Can you work these out from the model? Positions are in its coordinate system, mm. Face numbers are marked on the shaded views. A direction names the side the tool comes from. Give positions to 0.01 mm unless a question says otherwise; leave off trailing zeros. Loops run counter-clockwise (first coordinate to the right, second up) from the corner with the lowest first, then second, coordinate; pieces in that order, holes last. Notation, with made-up numbers: M 4,27 L 47,27 A32 cw 47,58 Z; hole C -18.5,21 d8. An arc over 180 degrees is marked long. Answer as a JSON object with one key per item and string values.
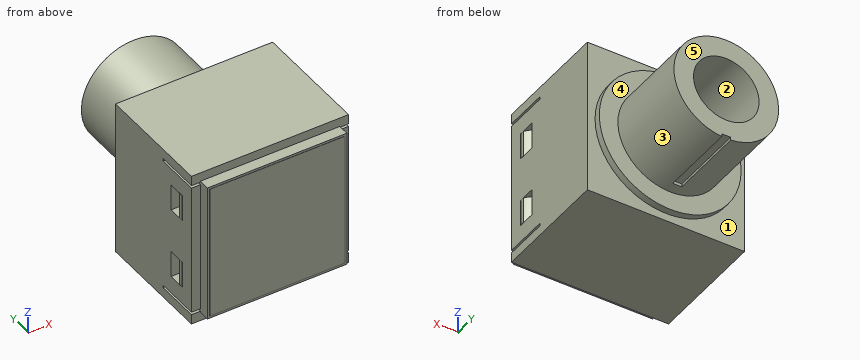
Autodesk Inventor part; units mm, degrees
ref_plane "body_to_dummy_XY" through (0, 0, 0) normal (0, 1, 0) x (1, 0, 0)
ref_plane "body_to_dummy_YZ" through (0, 0, 0) normal (1, 0, 0) x (0, 0, -1)
ref_plane "body_to_dummy_ZX" through (0, 0, 0) normal (0, 0, -1) x (0, 1, 0)
sketch "Sketch_1" plane through (0, 0, 0) normal (1, 0, 0) x (0, 1, 0)
  line L0 (0, 9.0043) -> (-15.5956, 9.0043)
  line L1 (-15.5956, 9.0043) -> (-15.5956, -9.0043)
  line L2 (-15.5956, -9.0043) -> (0, -9.0043)
  line L3 (0, -9.0043) -> (0, 9.0043)
extrude "Extrusion1" add sketch "Sketch_1" along normal mid plane 18.0086
sketch "Sketch_2" plane through (0, 0, 0) normal (0, 1, 0) x (-1, 0, 0)
  line L0 (12.2936, -12.2936) -> (12.2936, 12.2936)
  line L1 (12.2936, 12.2936) -> (-12.2936, 12.2936)
  line L2 (-12.2936, 12.2936) -> (-12.2936, -12.2936)
  line L3 (-12.2936, -12.2936) -> (12.2936, -12.2936)
  circle A0 centre (0, 0) radius 8.128
extrude "Extrusion2" cut sketch "Sketch_2" along normal mid plane 1.524
sketch "Sketch_3" plane through (0, -15.5956, 0) normal (0, 1, 0) x (1, 0, 0)
  line L0 (-11.5316, 11.5316) -> (-11.5316, -11.5316)
  line L1 (-11.5316, -11.5316) -> (11.5316, -11.5316)
  line L2 (11.5316, -11.5316) -> (11.5316, 11.5316)
  line L3 (11.5316, 11.5316) -> (-11.5316, 11.5316)
  line L4 (-7.9883, 7.9883) -> (-7.9883, -7.9883)
  line L5 (-7.9883, -7.9883) -> (7.9883, -7.9883)
  line L6 (7.9883, -7.9883) -> (7.9883, 7.9883)
  line L7 (7.9883, 7.9883) -> (-7.9883, 7.9883)
extrude "Extrusion3" cut sketch "Sketch_3" along normal mid plane 2.54
sketch "Sketch_4" plane through (0, -14.3256, 0) normal (0, 1, 0) x (1, 0, 0)
  line L0 (-12.446, 12.446) -> (-12.446, -12.446)
  line L1 (-12.446, -12.446) -> (12.446, -12.446)
  line L2 (12.446, -12.446) -> (12.446, 12.446)
  line L3 (12.446, 12.446) -> (-12.446, 12.446)
  line L4 (-11.5316, -7.5692) -> (-7.9883, -7.5692)
  line L5 (-7.9883, -7.5692) -> (-7.9883, -7.874)
  line L6 (-7.9883, -7.874) -> (-11.5316, -7.874)
  line L7 (-11.5316, -7.874) -> (-11.5316, -11.5316)
  line L8 (-11.5316, -11.5316) -> (11.5316, -11.5316)
  line L9 (11.5316, -11.5316) -> (11.5316, -7.874)
  line L10 (11.5316, -7.874) -> (7.9883, -7.874)
  line L11 (7.9883, -7.874) -> (7.9883, -7.5692)
  line L12 (7.9883, -7.5692) -> (11.5316, -7.5692)
  line L13 (11.5316, -7.5692) -> (11.5316, 7.5692)
  line L14 (11.5316, 7.5692) -> (7.9883, 7.5692)
  line L15 (7.9883, 7.5692) -> (7.9883, 7.874)
  line L16 (7.9883, 7.874) -> (11.5316, 7.874)
  line L17 (11.5316, 7.874) -> (11.5316, 11.5316)
  line L18 (11.5316, 11.5316) -> (-11.5316, 11.5316)
  line L19 (-11.5316, 11.5316) -> (-11.5316, 7.874)
  line L20 (-11.5316, 7.874) -> (-7.9883, 7.874)
  line L21 (-7.9883, 7.874) -> (-7.9883, 7.5692)
  line L22 (-7.9883, 7.5692) -> (-11.5316, 7.5692)
  line L23 (-11.5316, 7.5692) -> (-11.5316, -7.5692)
extrude "Extrusion4" cut sketch "Sketch_4" along normal mid plane 10.16
sketch "Sketch_5" plane through (0, -14.3256, 0) normal (0, 1, 0) x (1, 0, 0)
  line L0 (-7.7343, 7.7343) -> (-7.7343, -7.7343)
  line L1 (-7.7343, -7.7343) -> (7.7343, -7.7343)
  line L2 (7.7343, -7.7343) -> (7.7343, 7.7343)
  line L3 (7.7343, 7.7343) -> (-7.7343, 7.7343)
extrude "Extrusion5" add sketch "Sketch_5" against normal blind 1.2954
sketch "Sketch_6" plane through (9.0043, 0, 0) normal (1, 0, 0) x (0, 0, -1)
  line L0 (2.54, -10.668) -> (2.54, -12.7)
  line L1 (2.54, -12.7) -> (5.588, -12.7)
  line L2 (5.588, -12.7) -> (5.588, -10.668)
  line L3 (5.588, -10.668) -> (2.54, -10.668)
extrude "Extrusion6" cut sketch "Sketch_6" against normal blind 18.0086
sketch "Sketch_7" plane through (9.0043, 0, 0) normal (1, 0, 0) x (0, 0, -1)
  line L0 (-5.588, -10.668) -> (-5.588, -12.7)
  line L1 (-5.588, -12.7) -> (-2.54, -12.7)
  line L2 (-2.54, -12.7) -> (-2.54, -10.668)
  line L3 (-2.54, -10.668) -> (-5.588, -10.668)
extrude "Extrusion7" cut sketch "Sketch_7" against normal blind 18.0086
sketch "Sketch_8" plane through (0, 0, 4.064) normal (0, 0, 1) x (1, 0, 0)
  line L0 (-9.0043, -12.6492) -> (-8.9535, -12.6492)
  line L1 (-8.9535, -12.6492) -> (-8.9535, -12.7)
  line L2 (-8.9535, -12.7) -> (8.9535, -12.7)
  line L3 (8.9535, -12.7) -> (8.9535, -12.6492)
  line L4 (8.9535, -12.6492) -> (9.0043, -12.6492)
  line L5 (9.0043, -12.6492) -> (9.0043, -12.192)
  arc A0 (9.0043, -12.192) -> (7.7343, -11.176) centre (6.8661, -13.563) ccw
  line L6 (7.7343, -11.176) -> (7.7343, -10.668)
  line L7 (7.7343, -10.668) -> (-7.7343, -10.668)
  line L8 (-7.7343, -10.668) -> (-7.7343, -11.176)
  arc A1 (-7.7343, -11.176) -> (-9.0043, -12.192) centre (-6.8661, -13.563) ccw
  line L9 (-9.0043, -12.192) -> (-9.0043, -12.6492)
extrude "Extrusion8" add sketch "Sketch_8" along normal mid plane 2.9972
sketch "Sketch_9" plane through (0, 0, -4.064) normal (0, 0, 1) x (1, 0, 0)
  line L0 (-9.0043, -12.6492) -> (-8.9535, -12.6492)
  line L1 (-8.9535, -12.6492) -> (-8.9535, -12.7)
  line L2 (-8.9535, -12.7) -> (8.9535, -12.7)
  line L3 (8.9535, -12.7) -> (8.9535, -12.6492)
  line L4 (8.9535, -12.6492) -> (9.0043, -12.6492)
  line L5 (9.0043, -12.6492) -> (9.0043, -12.192)
  arc A0 (9.0043, -12.192) -> (7.7343, -11.176) centre (6.8661, -13.563) ccw
  line L6 (7.7343, -11.176) -> (7.7343, -10.668)
  line L7 (7.7343, -10.668) -> (-7.7343, -10.668)
  line L8 (-7.7343, -10.668) -> (-7.7343, -11.176)
  arc A1 (-7.7343, -11.176) -> (-9.0043, -12.192) centre (-6.8661, -13.563) ccw
  line L9 (-9.0043, -12.192) -> (-9.0043, -12.6492)
extrude "Extrusion9" add sketch "Sketch_9" along normal mid plane 2.9972
sketch "Sketch_11" plane through (0, 0, 0) normal (1, 0, 0) x (0, 1, 0)
  line L0 (0, 0) -> (10.0076, 0)
  line L1 (0, -3.7592) -> (0, -6)
  line L2 (0, -6) -> (10.0076, -6)
  line L3 (10.0076, -6) -> (10.0076, -3.7592)
  line L4 (10.0076, -3.7592) -> (0, -3.7592)
revolve "Revolution1" add sketch "Sketch_11" angle 360 about axis through (0, 0, 0) along (0, -1, 0)
thread "Thread1"
sketch "Sketch_15" plane through (0, 0, 0) normal (0, 1, 0) x (-1, 0, 0)
  line L0 (0.508, -5.6444) -> (-0.508, -5.6444)
  line L1 (-0.508, -5.6444) -> (-0.508, -6.4064)
  line L2 (-0.508, -6.4064) -> (0.508, -6.4064)
  line L3 (0.508, -6.4064) -> (0.508, -5.6444)
extrude "Extrusion10" cut sketch "Sketch_15" along normal blind 50.8
sketch "Sketch_18" plane through (0, 0, 0) normal (1, 0, 0) x (0, 1, 0)
  line L0 (0, 0) -> (1.27, 0)
  line L1 (1.27, 0) -> (1.27, -6)
  line L2 (1.27, -6) -> (0, -6)
  line L3 (0, -6) -> (0, 0)
  line L4 (0, 0) -> (1.27, 0)
revolve "Revolution2" add sketch "Sketch_18" angle 360 about axis through (0, 0, 0) along (0, -1, 0)
ref_plane "body_to_dummy_XY" through (0, 0, 0) normal (0, 1, 0) x (1, 0, 0)
ref_plane "body_to_dummy_YZ" through (0, 0, 0) normal (1, 0, 0) x (0, 0, -1)
ref_plane "body_to_dummy_ZX" through (0, 0, 0) normal (0, 0, -1) x (0, 1, 0)
ref_plane "body_to_hex_nut_XY" through (0, 0, 0) normal (0, 1, 0) x (1, 0, 0)
ref_plane "body_to_hex_nut_YZ" through (0, 0, 0) normal (1, 0, 0) x (0, 0, -1)
ref_plane "body_to_hex_nut_ZX" through (0, 0, 0) normal (0, 0, -1) x (0, 1, 0)
ref_plane "body_to_hex_nut_black_XY" through (0, 2.5146, 0) normal (0, 1, 0) x (1, 0, 0)
ref_plane "body_to_hex_nut_black_YZ" through (0, 2.5146, 0) normal (1, 0, 0) x (0, 0, -1)
ref_plane "body_to_hex_nut_black_ZX" through (0, 2.5146, 0) normal (0, 0, -1) x (0, 1, 0)
ref_plane "body_to_lockwasher_XY" through (0, 2.0066, 0) normal (0, 1, 0) x (1, 0, 0)
ref_plane "body_to_lockwasher_YZ" through (0, 2.0066, 0) normal (1, 0, 0) x (0, 0, -1)
ref_plane "body_to_lockwasher_ZX" through (0, 2.0066, 0) normal (0, 0, -1) x (0, 1, 0)
ref_plane "body_to_pins_XY" through (0, -15.5956, 0) normal (0, 1, 0) x (1, 0, 0)
ref_plane "body_to_pins_YZ" through (0, -15.5956, 0) normal (1, 0, 0) x (0, 0, -1)
ref_plane "body_to_pins_ZX" through (0, -15.5956, 0) normal (0, 0, -1) x (0, 1, 0)
ref_plane "body_to_toggles_XY" through (0, 10.0076, 0) normal (0, -1, 0) x (1, 0, 0)
ref_plane "body_to_toggles_YZ" through (0, 10.0076, 0) normal (1, 0, 0) x (0, 0, 1)
ref_plane "body_to_toggles_ZX" through (0, 10.0076, 0) normal (0, 0, 1) x (0, -1, 0)
properties part number "tl-cap"
1) Suppose I cut it at A-A, the plane y = 5.5. Write out the boundary of the cut face in (x, z), and give its area (3 significant figures).
Answer list:
{"outline": "M -0.51,-5.98 L -0.51,-5.64 L 0.51,-5.64 L 0.51,-5.98 A6 ccw long Z; hole C 0,0 d7.52", "area": "68.3 mm^2"}
2) Will this pin go through, and if not, where does the flat tip stop? pin 1 Ø2 at (x, z) = (-4.5, 6.5) entering from +Y.
Answer list:
{"pin 1": "y = 0"}
3) For the marked faces 4 and 5, which set-ups out of +Z, -Z, +X, -X, +Y, -Y let a thin tool reach every point of the face, with its end or its side?
Answer list:
{"face 4": "+Y", "face 5": "+Z, -Z, +X, -X, +Y"}
4) If we mould it in two halves opening along Z, with no side actions, what happens to the marked faces 1, 2 and 3? For each: +Z half, -Z half, draft (parallel to the pull), parting line (faces both ways), or undercut.
Answer list:
{"face 1": "draft", "face 2": "undercut", "face 3": "parting line"}
5) Suppose I cut it at C-C, the plane x = 6.75. Give the number of separate pieces and of enclosed holes in the cut face, and give its area (3 significant figures).
Answer list:
{"separate pieces": "1", "enclosed holes": "4", "area": "272 mm^2"}
6) Please list where these lines run through material, in increasing order: line 1 along X through (y, z) = (4.5, 0); line 2 along Y through (x, z) = (-7.75, -0.5); line 3 along Y through (x, z) = (-6.25, 7.5). Write a range as from..to.
Answer list:
{"line 1": "-6..-3.76, 3.76..6", "line 2": "-15.6..0", "line 3": "-15.62..-0.76"}
